Work out the finished part from the listing and answer in its coordinate system (mm). A direction names the side the tool comes from. Give positions to 0.01 mm unless a question says otherwise; leave off trailing zeros. Write each loop counter-clockwise with the first axis right and the second up, starting at its lowest first coordinate (ties: lowest second). Pieces come first, ordered by that corner, then holes. Notation, with made-up numbers: (-32, 52) - (-10, 52) arc R23 ccw to (-10, 79) - close; hole circle Ø11 at (44.25, 78.25). An arc over 180 degrees is marked (long way). Write item = value, one per line.
from build123d import *

# Parameters (mm, degrees)
F3_W     = 16.002
F3_H     = 12.3952
F4_DEPTH = 1.524
F1_R     = 3.81
F6_R     = 0.508
F7_W     = 1.016
F7_H     = 7.874
F2_DEPTH = 5.6896


with BuildPart() as f4:
    # F3 (on Front) → F4 (new body)
    with BuildSketch(Plane.XZ):
        Rectangle(F3_W, F3_H)
    extrude(amount=F4_DEPTH)

    # F0 (on Right) → F5 (revolve)
    with BuildSketch(Plane.YZ):
        Polygon((-42.799, 0), (-1.524, 0), (-1.524, 4.9276), (-21.209, 4.9276), (-32.131, 3.937), (-42.799, 3.937), align=None)
    revolve(axis=Axis((0, -21.3995, 0), (0, -1, 0)))

    # F1
    f1_edges = [f4.edges().sort_by_distance(p)[0] for p in [
        (0, -42.799, -3.937),
    ]]
    fillet(f1_edges, radius=F1_R)

    # F6
    f6_edges = [f4.edges().sort_by_distance(p)[0] for p in [
        (8.001, -0.762, 6.1976),
        (-8.001, -0.762, 6.1976),
        (-8.001, -0.762, -6.1976),
        (8.001, -0.762, -6.1976),
    ]]
    fillet(f6_edges, radius=F6_R)

    # F7 (on Top) → F2 (join)
    with BuildSketch(Plane.XY):
        with Locations((0, -15.621)):
            Rectangle(F7_W, F7_H)
    extrude(amount=F2_DEPTH)


solid = f4.part
1. Find section C-C, the plane y = -18. Give the vertices of the cut face in (x, z).
Solution:
outline = (-0.51, 4.9) arc R4.93 ccw (long way) to (0.51, 4.9) - (0.51, 5.69) - (-0.51, 5.69) - close
2. Straight lines are drawn through the part: line 1 (X direction, y = -16.5, z = 5.5); line 2 (Y direction, x = -3, z = -4.5); line 3 (X direction, y = -11.5, z = 0.25). For each, find the intervals that lie inside material, in ascending order.
Solution:
line_1 = -0.51 to 0.51
line_2 = -1.52 to 0
line_3 = -4.92 to 4.92
3. Find section A-A, the plane y = -3.5. Give the vertices of the cut face in (x, z).
Solution:
outline = circle Ø9.86 at (0, 0)
4. Given pin 1 (4 mm diameter, centred on x = 2, z = 2.5, fed in from -Y); pin 2 (0.5 mm diameter, centred on x = 0, y = -16, fed in from +Z); pin 3 (3 mm diameter, centred on x = 3, z = -2, fed in from -Y) (3 decimals), each flat-ended and moving along its own axis, determine where each tip first touches the part or whether it passes through.
Solution:
pin_1 = -42.64
pin_2 = 5.69
pin_3 = -42.245
5. Find section B-B, the plane x = -6.25. Give the vertices of the cut face in (y, z).
Solution:
outline = (-1.52, -6.2) - (0, -6.2) - (0, 6.2) - (-1.52, 6.2) - close
6. A tool of negligible diameter and unlimited length cuts with its end or side. For faces 1 (the flat face through (-8.001, -1, 0)), 2 (the flat face through (0, -16, 5.69)), 3 (the cylindrical face through (3.843, -35.608, -0.853)), from which of +Z, -Z, +X, -X, +Y, -Y can it reach the whole face along a straight path? Write none if from no direction.
Solution:
face_1 = +Z, -Z, -X, +Y, -Y
face_2 = +Z, +X, -X, -Y
face_3 = -Y
